Answer from the drawing. Dimensions are ordinates in mm from the lowest x, y and z of the part. Give positions to 0.01 mm unless a question says otherwise; leave off trailing zeros. Loops run counter-clockwise (first coordinate to the right, second up) from the corner with the lowest first, then second, coordinate; pieces in that order, holes last. Notation, with made-up numbers: (8.25, -20.75) - (42.25, -20.75) arc R18 cw to (42.25, 4.25) - close; hole circle Ø7 at (-6, 83.5). An arc over 180 degrees is marked (long way). Write each question's results on one line, items separated by ' | '. Start each with the question number.
Q1. Given pin 1 (3 mm diameter, centred on x = 15.5, z = 71, fed in from +Y); pin 2 (10 mm diameter, centred on x = 21.5, y = 69.5, fed in from +Z); pin 3 (8 mm diameter, centred on x = 5, z = 58.5, fed in from +Y), each flat-ended and moving along its own axis, determine where each tip first touches the part or whether it passes through.
Q2. Find the intervals of material crossed by line 1 (Z direction, x = 19.25, y = 62.5); line 2 (Y direction, x = 16, z = 51.5); line 3 (Y direction, x = 7.5, z = 70.5), in increasing order. Write a range as from..to.
Q3. Determine the mould class of the marked faces 1, 2 and 3 for opening direction Z: +Z half, -Z half, draft (parallel to the pull), parting line (faces both ways), or undercut.
Q4. The part is cut by section C-C, the plane x = 22. Write down the section's boundary in (y, z).
Q5. The part is cut by section A-A, the plane z = 62.5. Write down the section's boundary in (x, y).
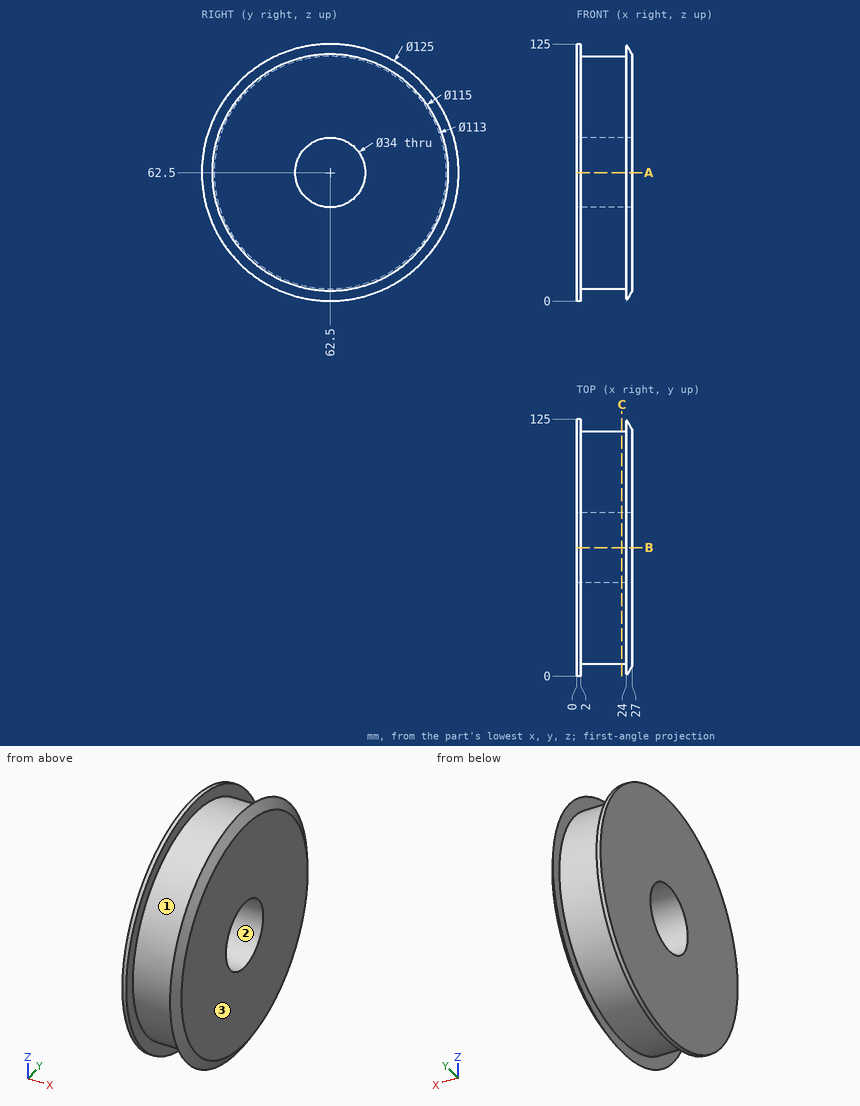
Check sheet entries:
1) pin 1: stops at y = 118.56 | pin 2: stops at z = 124.94 | pin 3: stops at y = 124.99
2) line 1: z = 6..45.5, 79.5..119 | line 2: y = 7.08..49.54, 75.46..117.92 | line 3: y = 6.57..47.5, 77.5..118.43
3) face 1: parting line | face 2: undercut | face 3: draft
4) outline: circle Ø113 at (62.5, 62.5); hole circle Ø34 at (62.5, 62.5)
5) outline: (0, 0) - (2, 0) - (2, 6) - (24, 6) - (24, 0) - (27, 5) - (27, 45.5) - (0, 45.5) - close; (0, 79.5) - (27, 79.5) - (27, 120) - (24, 125) - (24, 119) - (2, 119) - (2, 125) - (0, 125) - close
